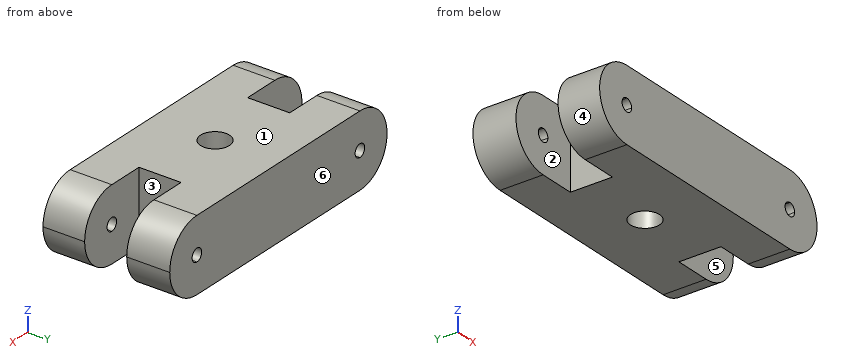
```python
from build123d import *

# Parameters (mm, degrees)
BOSS_EXTRUDE1_DEPTH    = 35
CUT_EXTRUDE1_START     = -20
CUT_EXTRUDE1_OUTLINE_W = 24.518111011
CUT_EXTRUDE1_OUTLINE_H = 11.618606297
CUT_EXTRUDE1_OUTLINE_R = 4
CUT_EXTRUDE1_DEPTH     = 20


# Read off the part's stored shape, not the designer's step: Cut-Extrude1
with BuildPart() as part:
    # Sketch1 → Boss-Extrude1 (new body)
    with BuildSketch(Plane(origin=(0, 0, 0), x_dir=(1, 0, 0), z_dir=(0, 1, 0))):
        with BuildLine():
            ThreePointArc((30, 10), (20, 0), (30, -10))
            Line((30, -10), (30, -1.75))
            ThreePointArc((30, -1.75), (28.25, 0), (30, 1.75))
            Line((30, 1.75), (30, 10))
        make_face()
        with BuildLine():
            Line((30, -1.75), (30, -10))
            ThreePointArc((30, -10), (37.071067812, -7.071067812), (40, 0))
            ThreePointArc((40, 0), (37.071067812, 7.071067812), (30, 10))
            Line((30, 10), (30, 1.75))
            ThreePointArc((30, 1.75), (31.237436867, 1.237436867), (31.75, 0))
            ThreePointArc((31.75, 0), (31.237436867, -1.237436867), (30, -1.75))
        make_face()
        with BuildLine():
            ThreePointArc((-30, 10), (-40, 0), (-30, -10))
            Line((-30, -10), (-30, -1.75))
            ThreePointArc((-30, -1.75), (-31.75, 0), (-30, 1.75))
            Line((-30, 1.75), (-30, 10))
        make_face()
        with BuildLine():
            Line((-30, -1.75), (-30, -10))
            ThreePointArc((-30, -10), (-22.928932188, -7.071067812), (-20, 0))
            ThreePointArc((-20, 0), (-22.928932188, 7.071067812), (-30, 10))
            Line((-30, 10), (-30, 1.75))
            ThreePointArc((-30, 1.75), (-28.762563133, 1.237436867), (-28.25, 0))
            ThreePointArc((-28.25, 0), (-28.762563133, -1.237436867), (-30, -1.75))
        make_face()
        with BuildLine():
            ThreePointArc((-20, 0), (-22.928932188, -7.071067812), (-30, -10))
            Line((-30, -10), (30, -10))
            ThreePointArc((30, -10), (20, 0), (30, 10))
            Line((30, 10), (-30, 10))
            ThreePointArc((-30, 10), (-22.928932188, 7.071067812), (-20, 0))
        make_face()
    extrude(amount=BOSS_EXTRUDE1_DEPTH)

    # Cut-Extrude1 outline → Cut-Extrude1 (cut)
    with BuildSketch(Plane(origin=(0, 0, -10), x_dir=(-1, 0, 0), z_dir=(0, 0, -1)).offset(CUT_EXTRUDE1_START)):
        with Locations((32.259055506, 17.309303148)):
            Rectangle(CUT_EXTRUDE1_OUTLINE_W, CUT_EXTRUDE1_OUTLINE_H)
        with Locations((-32.259055506, 17.309303148)):
            Rectangle(CUT_EXTRUDE1_OUTLINE_W, CUT_EXTRUDE1_OUTLINE_H)
        with Locations((0, 17.5)):
            Circle(CUT_EXTRUDE1_OUTLINE_R)
    extrude(amount=CUT_EXTRUDE1_DEPTH, mode=Mode.SUBTRACT)


solid = part.part
```
Geometry check sheet. Reference: the model listing, model coordinates, mm. Face numbers are marked on the shaded views. A direction names the side the tool comes from. Coordinates: 2 decimals unless noted, no trailing zeros. Write each loop counter-clockwise with the first axis right and the second up, starting at its lowest first coordinate (ties: lowest second). Pieces come first, ordered by that corner, then holes. Notation, with made-up numbers: (72, -16.5) -> (82, -16.5) arc R30 ccw to (82, 6.5) -> close; hole circle Ø1 at (0, 2.25). An arc over 180 degrees is marked (long way). Use CSV: the item, a comma, the result in double quotes. Start each with the question number.
Item 1: Cross-section at C-C, the plane z = -0.75. State how many separate pieces and enclosed holes the cut face has, plus the area to 3 significant figures.
Item 2: Set-up check for the marked faces 1, 2 and 3: record each of +Z, -Z, +X, -X, +Y, -Y from which the full face is reachable in a straight line by a thin tool's end or side.
Item 3: Mould release check, pull along Y, two halves, no side actions. Record for the marked faces 4, 5 and 6: released by +Y, released by -Y, zero draft, split by the parting line, or undercut.
Item 4: Cross-section at D-D, the plane z = 2.5. Record the cut outline in (x, y), plus the area to 3 significant figures.
Item 5: Cross-section at A-A, the plane y = 17.5. Record the cut outline in (x, z), plus the area to 3 significant figures.
Item 6: Cross-section at B-B, the plane x = -26.5. Record the cut outline in (y, z).
Item 7: Depth check by flat-ended pin: pin 1 Ø6.5 at (x, y) = (0, 17.5) entering from -Z; pin 2 Ø12 at (y, z) = (11, 7.5) entering from +X; pin 3 Ø2 at (y, z) = (5, 6) entering from +X; pin 4 Ø9.5 at (y, z) = (17.5, -2) entering from +X. Enter the tip coordinate at first touch or a pass-through.
Item 8: Thickness scan on line 1 (Y direction, x = 0, z = -0.5); line 2 (Y direction, x = -36, z = 5); line 3 (X direction, y = 3, z = 0.5). Record the ranges inside material, lowest first.
Answers:
1,separate pieces,"5"
1,enclosed holes,"1"
1,area,"2,140 mm^2"
2,face 1,"+Z, +X, -X, +Y, -Y"
2,face 2,"+Z, -Z, -X"
2,face 3,"+Z, -Z, +X"
3,face 4,"zero draft"
3,face 5,"undercut"
3,face 6,"released by +Y"
4,outline,"(-39.68, 0) -> (39.68, 0) -> (39.68, 11.5) -> (20, 11.5) -> (20, 23.12) -> (39.68, 23.12) -> (39.68, 35) -> (-39.68, 35) -> (-39.68, 23.12) -> (-20, 23.12) -> (-20, 11.5) -> (-39.68, 11.5) -> close; hole circle Ø8 at (0, 17.5)"
4,area,"2,270 mm^2"
5,outline,"(-20, -10) -> (-4, -10) -> (-4, 10) -> (-20, 10) -> close; (4, -10) -> (20, -10) -> (20, 10) -> (4, 10) -> close"
5,area,"640 mm^2"
6,outline,"(0, -10) -> (11.5, -10) -> (11.5, 10) -> (0, 10) -> close; (23.12, -10) -> (35, -10) -> (35, 10) -> (23.12, 10) -> close"
7,pin 1,"through"
7,pin 2,"x = 39.89"
7,pin 3,"x = 38.66"
7,pin 4,"x = 20"
8,line 1,"0 to 13.5, 21.5 to 35"
8,line 2,"0 to 11.5, 23.12 to 35"
8,line 3,"-39.99 to -31.68, -28.32 to 28.32, 31.68 to 39.99"
